Input: dimensioned drawing with shaded views. Units: mm. Origin: part minimum x, y, z. Round coordinates to 2 decimals unless told otherwise and drop trailing zeros. Loops run counter-clockwise (first coordinate to the right, second up) from the corner with the lowest first, then second, coordinate; pieces in that order, holes last. Notation, with made-up numbers: (-9, 68) - (49, 68) arc R26 cw to (49, 97) - close; hole circle Ø10 at (47, -27). An arc over 180 degrees is marked (long way). One line per question, with ' | ' between items.
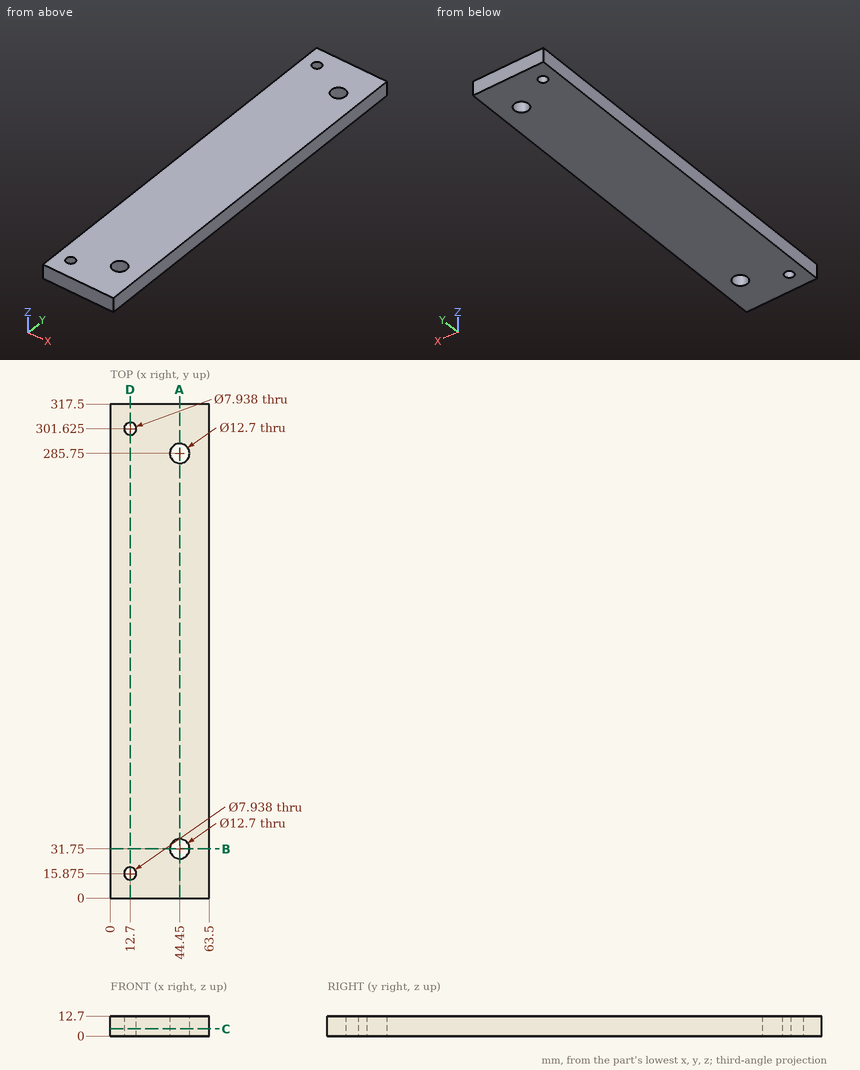
1. Section query A-A, the plane x = 44.45. Return loops of the section in (y, z), plus the area to 3 significant figures.
Worked out:
outline: (0, 0) - (25.4, 0) - (25.4, 12.7) - (0, 12.7) - close; (38.1, 0) - (279.4, 0) - (279.4, 12.7) - (38.1, 12.7) - close; (292.1, 0) - (317.5, 0) - (317.5, 12.7) - (292.1, 12.7) - close | area: 3,710 mm2
2. Material intervals for probe 1 along Y at (x, z) = (12.7, 8.25); probe 2 along Y at (x, z) = (44.45, 6); probe 3 along X at (y, z) = (285.75, 6.75), sorted ascending.
Worked out:
probe 1: y = 0 to 11.91, 19.84 to 297.66, 305.59 to 317.5 | probe 2: y = 0 to 25.4, 38.1 to 279.4, 292.1 to 317.5 | probe 3: x = 0 to 38.1, 50.8 to 63.5
3. Section query B-B, the plane y = 31.75. Return loops of the section in (x, z), plus the area to 3 significant figures.
Worked out:
outline: (0, 0) - (38.1, 0) - (38.1, 12.7) - (0, 12.7) - close; (50.8, 0) - (63.5, 0) - (63.5, 12.7) - (50.8, 12.7) - close | area: 645 mm2
4. Section query C-C, the plane z = 4.5. Give the number of separate pieces and of enclosed holes in the cut face, plus the area to 3 significant figures.
Worked out:
separate pieces: 1 | enclosed holes: 4 | area: 19,800 mm2
5. Section query D-D, the plane x = 12.7. Return loops of the section in (y, z), plus the area to 3 significant figures.
Worked out:
outline: (0, 0) - (11.91, 0) - (11.91, 12.7) - (0, 12.7) - close; (19.84, 0) - (297.66, 0) - (297.66, 12.7) - (19.84, 12.7) - close; (305.59, 0) - (317.5, 0) - (317.5, 12.7) - (305.59, 12.7) - close | area: 3,830 mm2
